Design review of the part shown in the three views and the two pictorial views. Dimensions are in mm from the part's minimum x, y and z. Give positions to 0.01 mm unless a question says otherwise; leave off trailing zeros. Order: outer loops, then holes, each group sorted by start corner. A loop starts at its lowest first (then second) coordinate and runs counter-clockwise, first axis right, second up.
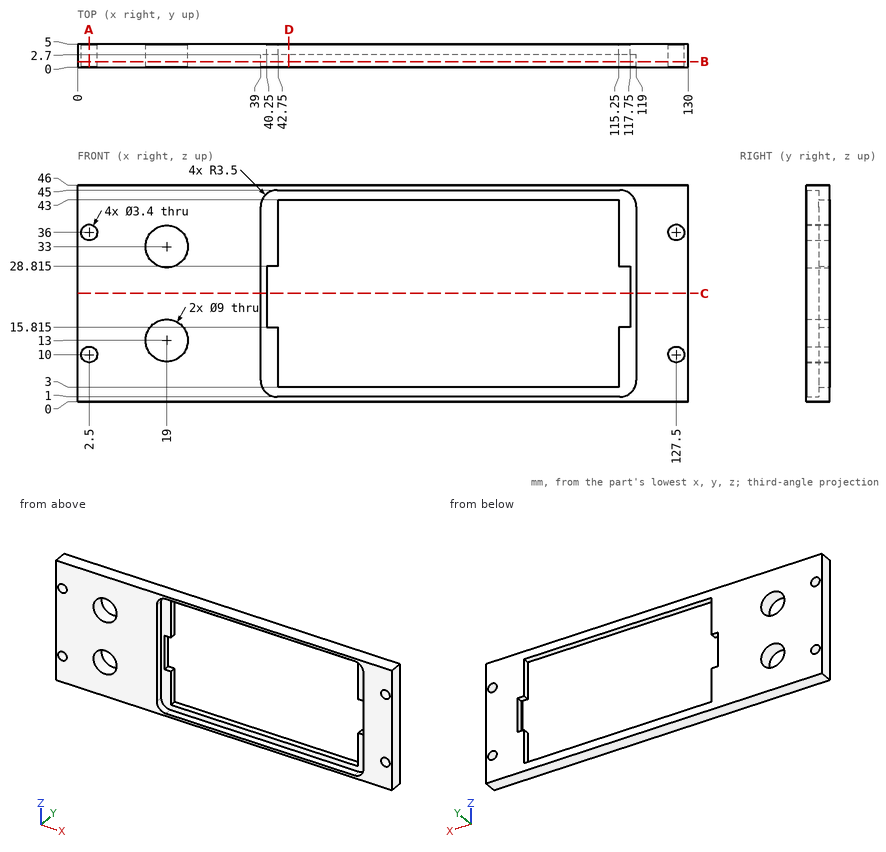
Item 1: Take a section at D-D (x = 45). Give the boundary of the cut face in (y, z).
Values found:
outline: (0, 0) - (5, 0) - (5, 3) - (2.7, 3) - (2.7, 1) - (0, 1) - close; (0, 45) - (2.7, 45) - (2.7, 43) - (5, 43) - (5, 46) - (0, 46) - close
Item 2: Take a section at C-C (z = 23). Give the boundary of the cut face in (x, y).
Values found:
outline: (0, 0) - (39, 0) - (39, 2.7) - (40.25, 2.7) - (40.25, 5) - (0, 5) - close; (117.75, 2.7) - (119, 2.7) - (119, 0) - (130, 0) - (130, 5) - (117.75, 5) - close
Item 3: Take a section at A-A (x = 2.5). Give the boundary of the cut face in (y, z).
Values found:
outline: (0, 0) - (5, 0) - (5, 8.3) - (0, 8.3) - close; (0, 11.7) - (5, 11.7) - (5, 34.3) - (0, 34.3) - close; (0, 37.7) - (5, 37.7) - (5, 46) - (0, 46) - close
Item 4: For line 1 (Z direction, x = 19, y = 3.05); line 2 (X direction, y = 1.9, z = 13); line 3 (X direction, y = 3.6, z = 13), list the stretches that pass through material, from the lowest coordinate up.
Values found:
line 1: z = 0 to 8.5, 17.5 to 28.5, 37.5 to 46
line 2: x = 0 to 14.5, 23.5 to 39, 119 to 130
line 3: x = 0 to 14.5, 23.5 to 42.75, 115.25 to 130
Item 5: Take a section at B-B (y = 1.25). Give the boundary of the cut face in (x, z), and give its area (3 significant figures).
Values found:
outline: (0, 0) - (130, 0) - (130, 46) - (0, 46) - close; hole circle Ø3.4 at (2.5, 10); hole circle Ø3.4 at (2.5, 36); hole circle Ø9 at (19, 13); hole circle Ø9 at (19, 33); hole (39, 4.5) arc R3.5 ccw to (42.5, 1) - (115.5, 1) arc R3.5 ccw to (119, 4.5) - (119, 41.5) arc R3.5 ccw to (115.5, 45) - (42.5, 45) arc R3.5 ccw to (39, 41.5) - close; hole circle Ø3.4 at (127.5, 10); hole circle Ø3.4 at (127.5, 36)
area: 2,310 mm2
